Part print with two shaded views. Sizes in mm from the minimum x, y, z corner. A direction names the side the tool comes from. Give positions to 0.01 mm unless a question says otherwise; leave off trailing zeros. Order: outer loops, then holes, each group sorted by start corner. A loop starts at its lowest first (then second) coordinate and runs counter-clockwise, first axis right, second up.
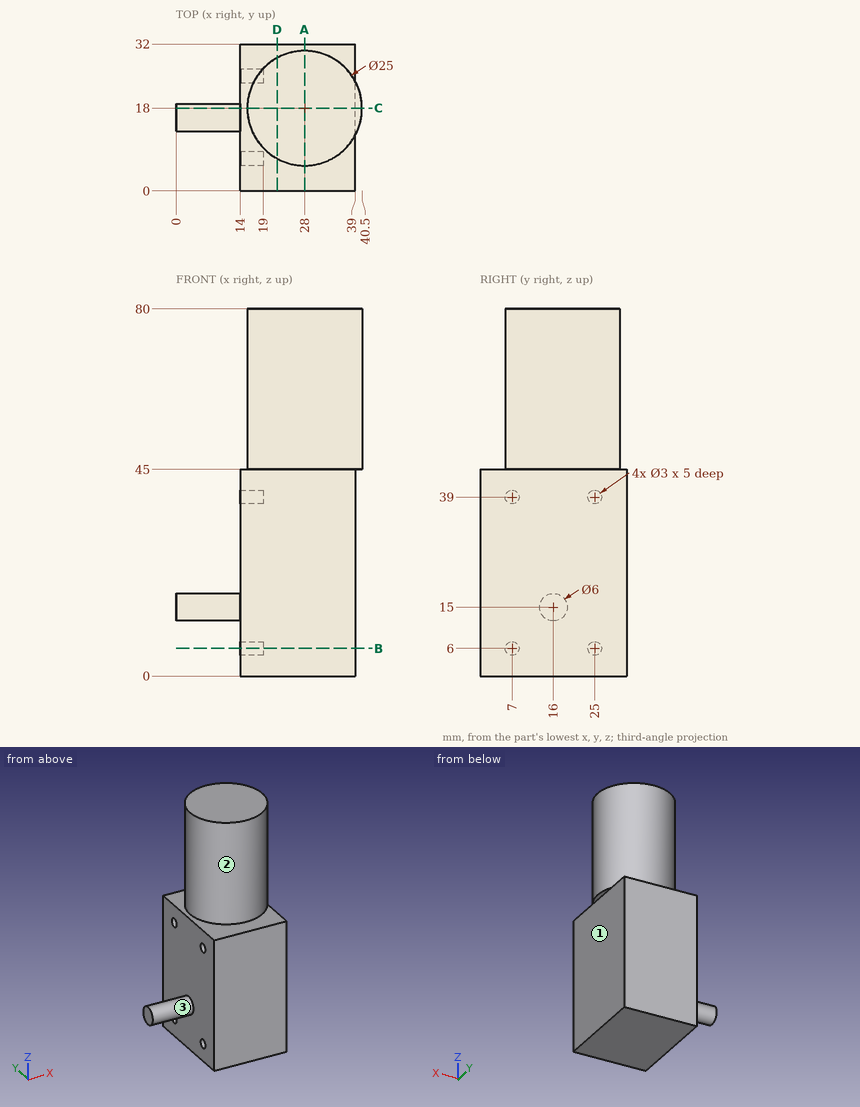
1. Saw through at A-A on x = 28. Give the cut face in (y, z).
2. Pin check, flat tips, straight feed: P1, Ø9.5, axis at y = 20.5, z = 30, coming from the -X side; P2, Ø8, axis at x = 10.5, y = 8, coming from the +Z side; P3, Ø10, axis at x = 6.5, y = 21, coming from the +Z side. Stop position of each tip, or through.
3. Saw through at B-B on z = 6. Give the cut face in (x, y).
4. 3-axis set-ups, long thin cutter, end or side, ignore diameter. For the marked faces 1, 2 and 3: which of +Z, -Z, +X, -X, +Y, -Y reach the whole face in a straight line?
5. Wall check: line 1 (Y direction, x = 15.35, z = 39); line 2 (Z direction, x = 16, y = 7); line 3 (Z direction, x = 32.5, y = 5.5). Give the ranges that are in metal, low to high.
6. Saw through at D-D on x = 22. Give the cut face in (y, z).
7. Saw through at C-C on y = 18. Give the cut face in (x, z).
Reported:
1. outline: (0, 0) - (32, 0) - (32, 45) - (30.5, 45) - (30.5, 80) - (5.5, 80) - (5.5, 45) - (0, 45) - close
2. P1: stops at x = 14
2. P2: stops at z = 45
2. P3: stops at z = 18
3. outline: (14, 0) - (39, 0) - (39, 32) - (14, 32) - (14, 26.5) - (19, 26.5) - (19, 23.5) - (14, 23.5) - (14, 8.5) - (19, 8.5) - (19, 5.5) - (14, 5.5) - close
4. face 1: -Z, +X, +Y, -Y
4. face 2: +Z
4. face 3: -X
5. line 1: y = 0 to 5.5, 8.5 to 23.5, 26.5 to 32
5. line 2: z = 0 to 4.5, 7.5 to 37.5, 40.5 to 45
5. line 3: z = 0 to 45
6. outline: (0, 0) - (32, 0) - (32, 45) - (28.97, 45) - (28.97, 80) - (7.03, 80) - (7.03, 45) - (0, 45) - close
7. outline: (0, 12.76) - (14, 12.76) - (14, 0) - (39, 0) - (39, 45) - (40.5, 45) - (40.5, 80) - (15.5, 80) - (15.5, 45) - (14, 45) - (14, 17.24) - (0, 17.24) - close
